```python
from build123d import *

# Parameters (mm, degrees)
PAD010_DEPTH = 0.25
PAD012_DEPTH = 0.25
PAD007_DEPTH = 3.5
PAD013_DEPTH = 0.25
PAD011_DEPTH = 0.25
PAD014_DEPTH = 0.2
SKETCH_W     = 10
SKETCH_H     = 6.5
PAD_DEPTH    = 4.8
FILLET_R     = 0.2


with BuildPart() as pad010:
    # Sketch011 → Pad010 (new body, symmetric)
    with BuildSketch(Plane.XZ.offset(1.59)):
        with BuildLine():
            Line((-2.54, 1.8), (-2.29, 1.8))
            Line((-2.29, 1.8), (-2.29, 0.4))
            ThreePointArc((-2.29, 0.4), (-2.246066, 0.293934), (-2.14, 0.25))
            Line((-1.4, 0.25), (-2.14, 0.25))
            Line((-1.4, 0), (-1.4, 0.25))
            Line((-1.4, 0), (-2.14, 0))
            ThreePointArc((-2.54, 0.4), (-2.422843, 0.117157), (-2.14, 0))
            Line((-2.54, 1.8), (-2.54, 0.4))
        make_face()
        with BuildLine():
            ThreePointArc((2.14, 0.25), (2.246066, 0.293934), (2.29, 0.4))
            Line((2.29, 1.8), (2.29, 0.4))
            Line((2.54, 1.8), (2.29, 1.8))
            Line((2.54, 0.4), (2.54, 1.8))
            ThreePointArc((2.139994, 0), (2.42284, 0.117155), (2.54, 0.4))
            Line((1.4, 0), (2.139994, 0))
            Line((1.4, 0.25), (1.4, 0))
            Line((2.14, 0.25), (1.4, 0.25))
        make_face()
    extrude(amount=PAD010_DEPTH, both=True)


with BuildPart() as pad012:
    # Sketch013 → Pad012 (new body, symmetric)
    with BuildSketch(Plane.XZ.offset(3.79)):
        with BuildLine():
            Line((-2.54, 1.8), (-2.29, 1.8))
            Line((-2.29, 1.8), (-2.29, 0.4))
            ThreePointArc((-2.29, 0.4), (-2.246066, 0.293934), (-2.14, 0.25))
            Line((-1.4, 0.25), (-2.14, 0.25))
            Line((-1.4, 0), (-1.4, 0.25))
            Line((-1.4, 0), (-2.14, 0))
            ThreePointArc((-2.54, 0.4), (-2.422843, 0.117157), (-2.14, 0))
            Line((-2.54, 1.8), (-2.54, 0.4))
        make_face()
        with BuildLine():
            ThreePointArc((2.14, 0.25), (2.246066, 0.293934), (2.29, 0.4))
            Line((2.29, 1.8), (2.29, 0.4))
            Line((2.54, 1.8), (2.29, 1.8))
            Line((2.54, 0.4), (2.54, 1.8))
            ThreePointArc((2.139994, 0), (2.42284, 0.117155), (2.54, 0.4))
            Line((1.4, 0), (2.139994, 0))
            Line((1.4, 0.25), (1.4, 0))
            Line((2.14, 0.25), (1.4, 0.25))
        make_face()
    extrude(amount=PAD012_DEPTH, both=True)


with BuildPart() as pad007:
    # Sketch009 → Pad007 (new body, symmetric)
    with BuildSketch(Plane.XZ):
        Polygon((-1.25, 0.25), (1.25, 0.25), (2.25, 1.05), (-2.25, 1.05), align=None)
    extrude(amount=PAD007_DEPTH, both=True)


with BuildPart() as pad013:
    # Sketch014 → Pad013 (new body, symmetric)
    with BuildSketch(Plane.XZ.offset(-0.61)):
        with BuildLine():
            Line((-2.54, 1.8), (-2.29, 1.8))
            Line((-2.29, 1.8), (-2.29, 0.4))
            ThreePointArc((-2.29, 0.4), (-2.246066, 0.293934), (-2.14, 0.25))
            Line((-1.4, 0.25), (-2.14, 0.25))
            Line((-1.4, 0), (-1.4, 0.25))
            Line((-1.4, 0), (-2.14, 0))
            ThreePointArc((-2.54, 0.4), (-2.422843, 0.117157), (-2.14, 0))
            Line((-2.54, 1.8), (-2.54, 0.4))
        make_face()
        with BuildLine():
            ThreePointArc((2.14, 0.25), (2.246066, 0.293934), (2.29, 0.4))
            Line((2.29, 1.8), (2.29, 0.4))
            Line((2.54, 1.8), (2.29, 1.8))
            Line((2.54, 0.4), (2.54, 1.8))
            ThreePointArc((2.139994, 0), (2.42284, 0.117155), (2.54, 0.4))
            Line((1.4, 0), (2.139994, 0))
            Line((1.4, 0.25), (1.4, 0))
            Line((2.14, 0.25), (1.4, 0.25))
        make_face()
    extrude(amount=PAD013_DEPTH, both=True)


with BuildPart() as pad011:
    # Sketch012 → Pad011 (new body, symmetric)
    with BuildSketch(Plane.XZ.offset(-3.81)):
        with BuildLine():
            Line((-2.54, 1.8), (-2.29, 1.8))
            Line((-2.29, 1.8), (-2.29, 0.4))
            ThreePointArc((-2.29, 0.4), (-2.246066, 0.293934), (-2.14, 0.25))
            Line((-1.4, 0.25), (-2.14, 0.25))
            Line((-1.4, 0), (-1.4, 0.25))
            Line((-1.4, 0), (-2.14, 0))
            ThreePointArc((-2.54, 0.4), (-2.422843, 0.117157), (-2.14, 0))
            Line((-2.54, 1.8), (-2.54, 0.4))
        make_face()
        with BuildLine():
            ThreePointArc((2.14, 0.25), (2.246066, 0.293934), (2.29, 0.4))
            Line((2.29, 1.8), (2.29, 0.4))
            Line((2.54, 1.8), (2.29, 1.8))
            Line((2.54, 0.4), (2.54, 1.8))
            ThreePointArc((2.139994, 0), (2.42284, 0.117155), (2.54, 0.4))
            Line((1.4, 0), (2.139994, 0))
            Line((1.4, 0.25), (1.4, 0))
            Line((2.14, 0.25), (1.4, 0.25))
        make_face()
    extrude(amount=PAD011_DEPTH, both=True)


with BuildPart() as pad014:
    # Sketch001 → Pad014 (new body)
    with BuildSketch(Plane(origin=(0, 0, 5.6), x_dir=(0, -1, 0), z_dir=(0, 0, 1))):
        with BuildLine():
            Line((-3.8, -1.8), (-3.8, 2.2))
            ThreePointArc((-3.8, 2.2), (-4, 2.4), (-4.2, 2.2))
            Line((-4.2, 2.2), (-4.2, -1.8))
            ThreePointArc((-4.2, -1.8), (-4, -2), (-3.8, -1.8))
        make_face()
    extrude(amount=PAD014_DEPTH)


with BuildPart() as obj1:
    # Sketch → Pad (new body)
    with BuildSketch(Plane(origin=(0, 0, 0.85), x_dir=(0, -1, 0), z_dir=(0, 0, 1))):
        with Locations((0, 0.25)):
            Rectangle(SKETCH_W, SKETCH_H)
    extrude(amount=PAD_DEPTH)

    # Fillet
    fillet_edges = [obj1.edges().sort_by_distance(p)[0] for p in [
        (-3, 0, 5.65),
        (0.25, -5, 5.65),
        (3.5, 0, 5.65),
        (0.25, 5, 5.65),
    ]]
    fillet(fillet_edges, radius=FILLET_R)

    add(pad010.part)
    add(pad012.part)
    add(pad007.part)
    add(pad013.part)
    add(pad011.part)
    add(pad014.part)


solid = obj1.part
```
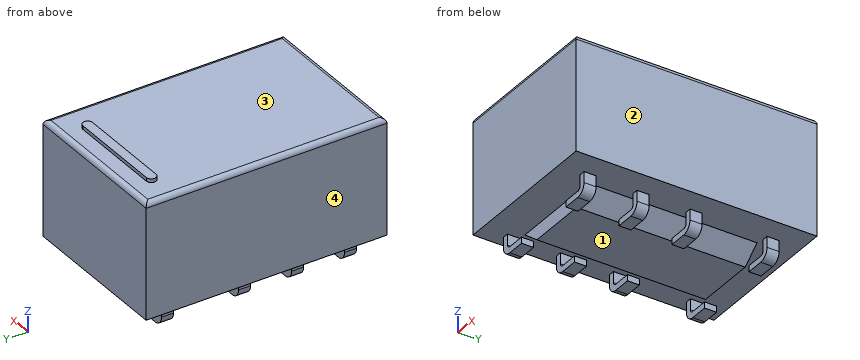
Geometry check sheet. Reference: the model listing, model coordinates, mm. Face numbers are marked on the shaded views. Give positions to 0.01 mm unless a question says otherwise; leave off trailing zeros. Write each loop counter-clockwise with the first axis right and the second up, starting at its lowest first coordinate (ties: lowest second). Pieces come first, ordered by that corner, then holes. Notation, with made-up numbers: (51.5, -21) -> (67.5, -21) arc R32 ccw to (67.5, 14) -> close; hole circle Ø2 at (64, 24). An arc over 180 degrees is marked (long way). Use one line per item in the form item = value.
Item 1: Depth check by flat-ended pin: pin 1 Ø0.5 at (x, z) = (-0.5, 0.5) entering from +Y. Enter the tip coordinate at first touch or a pass-through.
Results list:
pin_1 = 3.5
Item 2: Scan lines: line 1 (Z direction, x = -0.5, y = -2.5); line 2 (Z direction, x = -2.5, y = 4.75); line 3 (Y direction, x = 0.75, z = 0.7). Record each from-to range of solid material in increasing order.
Results list:
line_1 = 0.25 to 5.65
line_2 = 0.85 to 5.65
line_3 = -3.5 to 3.5
Item 3: Sectioned sample at C-C on y = -4.5. Enter the section's corners in (x, z).
Results list:
outline = (-3, 0.85) -> (3.5, 0.85) -> (3.5, 5.45) arc R0.2 ccw to (3.3, 5.65) -> (-2.8, 5.65) arc R0.2 ccw to (-3, 5.45) -> close
Item 4: Sectioned sample at B-B on x = 3. Enter the section's corners in (y, z).
Results list:
outline = (-5, 0.85) -> (5, 0.85) -> (5, 5.45) arc R0.2 ccw to (4.8, 5.65) -> (-4.8, 5.65) arc R0.2 ccw to (-5, 5.45) -> close
Item 5: Sectioned sample at A-A on y = -0.5. Enter the section's corners in (x, z), plus the area to 3 significant figures.
Results list:
outline = (-3, 0.85) -> (-2, 0.85) -> (-1.25, 0.25) -> (1.25, 0.25) -> (2, 0.85) -> (3.5, 0.85) -> (3.5, 5.45) arc R0.2 ccw to (3.3, 5.65) -> (-2.8, 5.65) arc R0.2 ccw to (-3, 5.45) -> close
area = 33.1 mm2
Item 6: Mould release check, pull along X, two halves, no side actions. Record for the marked faces 1, 2, 3 and 4: released by +X, released by -X, zero draft, split by the parting line, or undercut.
Results list:
face_1 = undercut
face_2 = released by +X
face_3 = zero draft
face_4 = released by -X
